Source: three-view drawing plus pictorial views. Frame: mm from the lowest corner of the part. A direction names the side the tool comes from. Round coordinates to 2 decimals unless told otherwise and drop trailing zeros. Order: outer loops, then holes, each group sorted by start corner. A loop starts at its lowest first (then second) coordinate and runs counter-clockwise, first axis right, second up. Notation, with made-up numbers: (-38.5, -0.75) -> (13.5, -0.75) arc R20 cw to (13.5, 15.25) -> close; hole circle Ø7 at (84.25, -25.5). An arc over 180 degrees is marked (long way). Answer as CSV lines item,"result". Start each with the question number.
1) Line query: L1, parallel to Y at x = 13.5, z = 5; L2, parallel to X at y = 7.5, z = 8; L3, parallel to Z at x = 12.5, y = 4.5 (1 decimal). Output: solid intervals per line, ascending.
2) Access query for the marked faces 1 and 2. Directions: +Z, -Z, +X, -X, +Y, -Y. A direction counts if a zero-diameter tool reaches every point of the face in a straight line with its end or side. Return the directions, or none.
3) Section query A-A, the plane z = 9. Output: boundary loops of the cut face in (x, y).
4) Section query D-D, the plane z = 5. Output: boundary loops of the cut face in (x, y).
5) Section query B-B, the plane y = 5. Output: boundary loops of the cut face in (x, z).
6) Section query C-C, the plane x = 4. Output: boundary loops of the cut face in (y, z), and give its area (3 significant figures).
7) First-contact query: P1, Ø1, axis at x = 14.5, z = 4, coming from the -Y side (1 decimal); P2, Ø5, axis at x = 4.5, z = 7, coming from the -Y side; P3, Ø1.6, axis at x = 14, z = 4, coming from the +Y side. Flat tips, straight axial feed; report the tip coordinate or a pass-through.
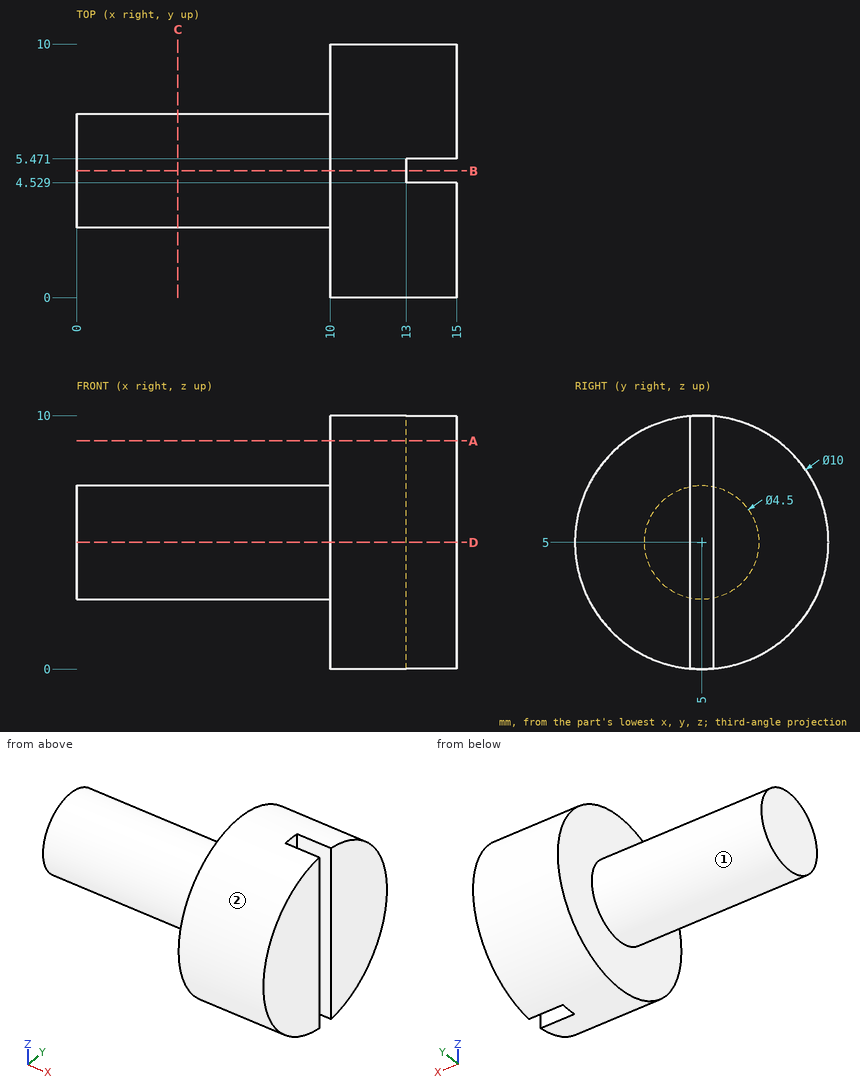
Findings:
1,L1,"y = 0 to 4.53, 5.47 to 10"
1,L2,"x = 10 to 15"
1,L3,"z = 0 to 10"
2,face 1,"-X"
2,face 2,"+X, -X"
3,outline,"(10, 2) -> (15, 2) -> (15, 4.53) -> (13, 4.53) -> (13, 5.47) -> (15, 5.47) -> (15, 8) -> (10, 8) -> close"
4,outline,"(0, 2.75) -> (10, 2.75) -> (10, 0) -> (15, 0) -> (15, 4.53) -> (13, 4.53) -> (13, 5.47) -> (15, 5.47) -> (15, 10) -> (10, 10) -> (10, 7.25) -> (0, 7.25) -> close"
5,outline,"(0, 2.75) -> (10, 2.75) -> (10, 0) -> (13, 0) -> (13, 10) -> (10, 10) -> (10, 7.25) -> (0, 7.25) -> close"
6,outline,"circle Ø4.5 at (5, 5)"
6,area,"15.9 mm^2"
7,P1,"stops at y = 0"
7,P2,"stops at y = 2.75"
7,P3,"stops at y = 10"
